from build123d import *

# Parameters (mm, degrees)
F0_R     = 80
F1_DEPTH = 5
F2_R     = 37.5
F3_DEPTH = 5.001
F4_R     = 80
F4_R_2   = 77.5
F5_DEPTH = 3


with BuildPart() as f1:
    # F0 (on Top) → F1 (new body)
    with BuildSketch(Plane.XY):
        Circle(F0_R)
    extrude(amount=F1_DEPTH)

    # F2 (on face) → F3 (cut, through all)
    with BuildSketch(Plane.XY.offset(5)):
        Circle(F2_R)
    extrude(amount=-F3_DEPTH, mode=Mode.SUBTRACT)

    # F4 (on face) → F5 (join)
    with BuildSketch(Plane.XY.offset(5)):
        Circle(F4_R)
        Circle(F4_R_2, mode=Mode.SUBTRACT)
    extrude(amount=F5_DEPTH)


solid = f1.part
Could you check a few things on this model? Use its own coordinates, in mm. A direction names the side the tool comes from. Round coordinates to 2 decimals unless told otherwise and drop trailing zeros. Order: outer loops, then holes, each group sorted by start corner. A loop starts at its lowest first (then second) coordinate and runs counter-clockwise, first axis right, second up. Notation, with made-up numbers: M -27.5,20.5 L -6.5,20.5 A17 ccw -6.5,36.5 Z; hole C 83.5,89 d7. An arc over 180 degrees is marked long. One line per item, written item: value.
(1) If we mould it in two halves opening along Y, with no side actions, what happens to faces 3 (the flat face through (17, -34, 0)), 4 (the flat face through (33.4, 18.3, 5)), 5 (the cylindrical face through (-17.34, -78.1, 3.94))? For each: released by +Y, released by -Y, zero draft, split by the parting line, or undercut.
Ans:
face 3: zero draft
face 4: undercut
face 5: split by the parting line
(2) Imagine slicing it at D-D (z = 2.75). Write out the boundary of the cut face in (x, y), and give its area (3 significant figures).
Ans:
outline: C 0,0 d160; hole C 0,0 d75
area: 15,700 mm^2
(3) Imagine slicing it at C-C (y = 54). Write out the boundary of the cut face in (x, z).
Ans:
outline: M -59.03,0 L 59.03,0 L 59.03,8 L 55.59,8 L 55.59,5 L -55.59,5 L -55.59,8 L -59.03,8 Z
(4) I need wall thicknesses on line 1 along Y through (x, z) = (0, 6.8); line 2 along Y through (x, z) = (0, 2.9); line 3 along Z through (x, y) = (-59, 28). Which ranges of each line are inside material? Lowest first, please. Write a range as from..to.
Ans:
line 1: y = -80..-77.5, 77.5..80
line 2: y = -80..-37.5, 37.5..80
line 3: z = 0..5
(5) I'm going to push flat-ended pins straight in: P1, Ø3, axis at y = 41.5, z = 4, coming from the -X side; P2, Ø2, axis at x = -31, y = -31.5, coming from the +Z side; P3, Ø2, axis at y = 61.5, z = 6, coming from the +X side. Where does each tip first touch, or does it pass through?
Ans:
P1: stops at x = -69.28
P2: stops at z = 5
P3: stops at x = 52.34
(6) Imagine slicing it at A-A (y = 0). Write out the boundary of the cut face in (x, z).
Ans:
outline: M -80,0 L -37.5,0 L -37.5,5 L -77.5,5 L -77.5,8 L -80,8 Z; M 37.5,0 L 80,0 L 80,8 L 77.5,8 L 77.5,5 L 37.5,5 Z
(7) Which directions (+Z, -Z, +X, -X, +Y, -Y) give clear straight access to the entire face, cutting with the end or side of a thin tool? Please do faces 1 (the cylindrical face through (-16.8, -75.657, 6.479)), 2 (the cylindrical face through (-4.88, 37.18, 2.54)).
Ans:
face 1: +Z
face 2: +Z, -Z
